Check sheet for the modelled part. Datum: model origin and axes. Units: mm. Face numbers are marked on the shaded views. Give positions to 0.01 mm unless a question says otherwise; leave off trailing zeros. Write each loop counter-clockwise with the first axis right and the second up, starting at its lowest first coordinate (ties: lowest second). Pieces come first, ordered by that corner, then holes. Notation, with made-up numbers: M 37.25,82 L 94.25,82 A21 ccw 94.25,116 Z; hole C 86.5,50 d8. An arc over 180 degrees is marked long. Write item = value, one per line. Start each with the question number.
1) Scan lines: L1, parallel to Z at x = 10, y = 0 (3 decimals); L2, parallel to Y at x = 2, z = -38; L3, parallel to Z at x = -4.5, y = 0 (3 decimals). Record each from-to range of solid material in increasing order.
2) Sectioned sample at C-C, the plane x = 9. Record the cut outline in (y, z) (3 decimals).
3) Sectioned sample at B-B, the plane y = 0. Count the separate pieces of the cut face and the enclosed holes in it, then the cut area to 3 significant figures.
4) Gauge pin test, flat ends, axial feed: pin 1 (7.5 mm diameter, centred on y = 0, z = -12.7, fed in from +X) (3 decimals); pin 2 (14 mm diameter, centred on y = 0, z = 41, fed in from -X) (3 decimals); pin 3 (14.5 mm diameter, centred on x = 9, y = 10, fed in from -Z). Record the tip position at first contact, or that the pin passes through.
5) Draft check along Z on the marked faces 1, 2, 3 and 4. Enter one of: pulls with the +Z half, pulls with the -Z half, needs draft (parallel to the pull), parting line crosses it, or undercut.
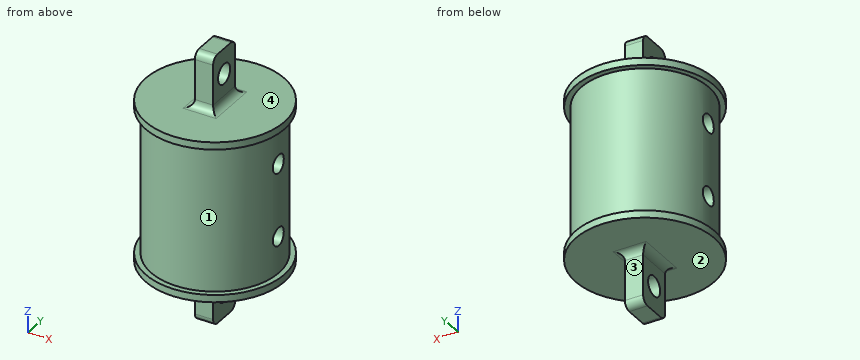
from build123d import *

# Parameters (mm, degrees)
SKETCH1_R               = 22.225
BOSS_EXTRUDE1_DEPTH     = 25.4
SKETCH2_R               = 24.13
BOSS_EXTRUDE2_DEPTH     = 2.54
SKETCH3_W               = 6.35
SKETCH3_H               = 12.7
BOSS_EXTRUDE3_DEPTH     = 19.05
SKETCH4_R               = 3.4925
CUT_EXTRUDE1_DEPTH      = 28.305
FILLET1_R               = 2.54
FILLET1_OF_MIRROR1_R    = 2.54
SKETCH5_R               = 3.175
CUT_EXTRUDE2_DEPTH      = 25.13
CUT_EXTRUDE2_DEPTH_BACK = 25.13


with BuildPart() as part:
    # Sketch1 → Boss-Extrude1 (new body, symmetric)
    with BuildSketch(Plane.XY):
        Circle(SKETCH1_R)
    extrude(amount=BOSS_EXTRUDE1_DEPTH, both=True)

    # Sketch2 → Boss-Extrude2 (add)
    with BuildSketch(Plane.XY.offset(25.4)):
        Circle(SKETCH2_R)
    boss_extrude2 = extrude(amount=BOSS_EXTRUDE2_DEPTH)

    # Sketch3 → Boss-Extrude3 (add)
    with BuildSketch(Plane.XY.offset(27.94)):
        Rectangle(SKETCH3_W, SKETCH3_H)
    boss_extrude3 = extrude(amount=BOSS_EXTRUDE3_DEPTH)

    # Sketch4 → Cut-Extrude1 (cut, through all)
    with BuildSketch(Plane(origin=(3.175, 0, 0), x_dir=(0, 0, -1), z_dir=(1, 0, 0))):
        with Locations((-38.1, 0)):
            Circle(SKETCH4_R)
    cut_extrude1 = extrude(amount=-CUT_EXTRUDE1_DEPTH, mode=Mode.SUBTRACT)

    # Fillet1
    fillet1_edges = [part.edges().sort_by_distance(p)[0] for p in [
        (3.175, 0, 27.94),
        (0, 6.35, 27.94),
        (-3.175, 0, 27.94),
        (0, -6.35, 27.94),
        (0, 6.35, 46.99),
        (0, -6.35, 46.99),
    ]]
    fillet(fillet1_edges, radius=FILLET1_R)

    # Mirror1: Boss-Extrude2, Boss-Extrude3, Cut-Extrude1 across plane
    add(boss_extrude2.mirror(Plane.XY))
    add(boss_extrude3.mirror(Plane.XY))
    add(cut_extrude1.mirror(Plane.XY), mode=Mode.SUBTRACT)

    # Fillet1 of Mirror1
    fillet1_of_mirror1_edges = [part.edges().sort_by_distance(p)[0] for p in [
        (3.175, 0, -27.94),
        (0, 6.35, -27.94),
        (-3.175, 0, -27.94),
        (0, -6.35, -27.94),
        (0, 6.35, -46.99),
        (0, -6.35, -46.99),
    ]]
    fillet(fillet1_of_mirror1_edges, radius=FILLET1_OF_MIRROR1_R)

    # Sketch5 → Cut-Extrude2 (cut, two sides)
    with BuildSketch(Plane(origin=(0, 0, 0), x_dir=(0, 0, -1), z_dir=(1, 0, 0))) as cut_extrude2_sk:
        with Locations((-12.7, 0)):
            Circle(SKETCH5_R)
        with Locations((12.7, 0)):
            Circle(SKETCH5_R)
    extrude(amount=CUT_EXTRUDE2_DEPTH, mode=Mode.SUBTRACT)
    extrude(cut_extrude2_sk.sketch, amount=-CUT_EXTRUDE2_DEPTH_BACK, mode=Mode.SUBTRACT)


solid = part.part
Data:
q1.L1 = -27.94 to -15.875, -9.525 to 9.525, 15.875 to 27.94
q1.L2 = -6.35 to -3.49, 3.49 to 6.35
q1.L3 = -28.249 to -15.875, -9.525 to 9.525, 15.875 to 28.249
q2.outline = M -22.389,-27.94 L 22.389,-27.94 L 22.389,-25.4 L 20.321,-25.4 L 20.321,25.4 L 22.389,25.4 L 22.389,27.94 L -22.389,27.94 L -22.389,25.4 L -20.321,25.4 L -20.321,-25.4 L -22.389,-25.4 Z; hole C 0,-12.7 d6.35; hole C 0,12.7 d6.35
q3.separate_pieces = 5
q3.enclosed_holes = 0
q3.area = 2,100 mm2
q4.pin_1 = 22.225
q4.pin_2 = -3.175
q4.pin_3 = -46.17
q5.face_1 = undercut
q5.face_2 = pulls with the -Z half
q5.face_3 = needs draft
q5.face_4 = pulls with the +Z half
